Autodesk Inventor part; units mm, degrees
ref_plane "YZ Plane" through (0, 0, 0) normal (1, 0, 0) x (0, 1, 0)
ref_plane "XZ Plane" through (0, 0, 0) normal (0, 1, 0) x (-1, 0, 0)
ref_plane "XY Plane" through (0, 0, 0) normal (0, 0, 1) x (1, 0, 0)
sketch "Szkic1" plane through (0, 0, 0) normal (0, 1, 0) x (-1, 0, 0)
  circle A0 centre (0, 0) radius 5.7
  dimension "d0" = 11.4
extrude "Wyciągnięcie proste1" add sketch "Szkic1" along normal blind 90
sketch "Szkic5" plane through (0, 90, 0) normal (0, 1, 0) x (1, 0, 0)
  point P0 (0, 0)
  point P1 (0, 0)
hole "Otwór2" at (0, 90, 0) direction (0, -1, 0) diameter 6 depth 35 tip angle 120
chamfer "Faza1" distance 1.5 angle 45 2 edges at (5.7, 90, 0) (5.7, 0, 0)
sketch "Szkic6" plane through (0, 0, 0) normal (0, 0, 1) x (1, 0, 0)
  circle A0 centre (0, 5) radius 2.5
  point P0 (0, 0)
  dimension "d20" = 5
extrude "Wyciągnięcie proste2" cut sketch "Szkic6" along normal mid plane 30
properties material "Stal nierdzewna"
Build history of the part. All positions in model axes, mm. Round coordinates to 2 decimals unless told otherwise and drop trailing zeros. Write each loop counter-clockwise with the first axis right and the second up, starting at its lowest first coordinate (ties: lowest second). Pieces come first, ordered by that corner, then holes. Notation, with made-up numbers: (23, -19.5) -> (73, -19.5) arc R22 cw to (73, 1.5) -> close; hole circle Ø10 at (61.5, 37.5). An arc over 180 degrees is marked (long way). Use one line per item in the form item = value.
Q1. Drop a flat-ended pin along its axis: P1, Ø2, axis at y = 21.5, z = -4, coming from the +X side. Give the stop position or say it passes through.
Conclusion:
P1 = 4.85
Q2. Band-saw the part on C-C, the plane y = 5. Write the cut outline in (x, z).
Conclusion:
outline = (-2.5, -5.12) -> (-2.5, 5.12) arc R5.7 ccw to start; (2.5, -5.12) arc R5.7 ccw to (2.5, 5.12) -> close
Q3. Drill centre line: L1, parallel to Y at x = -0.25, z = -4. Where is it in solid material? Low to high.
Conclusion:
L1 = 0 to 2.51, 7.49 to 90
Q4. Two-plate mould, pull along Z, no slides. Class faces 1 (the conical face through (-0.51, 53.57, -0.11)), 2 (the cylindrical face through (0, 72, -3)), 3 (the cylindrical face through (2.385, 5.751, 0.08)), 4 (the cylindrical face through (-5.265, 44.391, 2.183)): released by +Z, released by -Z, zero draft, split by the parting line, or undercut.
Conclusion:
face_1 = undercut
face_2 = undercut
face_3 = zero draft
face_4 = split by the parting line
Q5. Band-saw the part on A-A, the plane y = 83.5. Write the cut outline in (x, z).
Conclusion:
outline = circle Ø11.4 at (0, 0); hole circle Ø6 at (0, 0)
Q6. Band-saw the part on B-B, the plane y = 14. Write the cut outline in (x, z), then the cut area to 3 significant figures.
Conclusion:
outline = circle Ø11.4 at (0, 0)
area = 102 mm²
